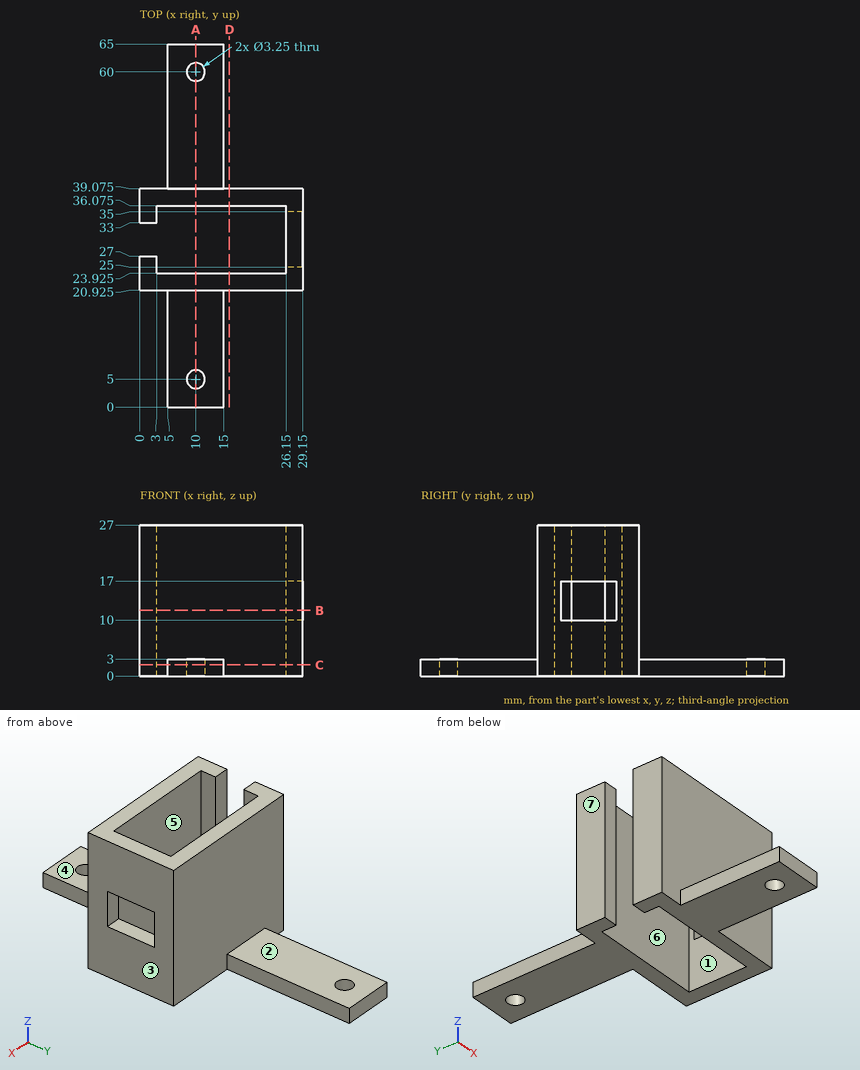
Input: dimensioned drawing with shaded views. Units: mm. Origin: part minimum x, y, z. A direction names the side the tool comes from. Coordinates: 2 decimals unless noted, no trailing zeros. Order: outer loops, then holes, each group sorted by start corner. A loop starts at its lowest first (then second) coordinate and runs counter-clockwise, first axis right, second up.
1. Cut plane B-B, the plane z = 11.75. Return loops of the section in (x, y) (3 decimals), plus the area to 3 significant figures.
Checked values:
outline: (0, 20.925) - (29.15, 20.925) - (29.15, 25) - (26.15, 25) - (26.15, 23.925) - (3, 23.925) - (3, 27) - (0, 27) - close; (0, 33) - (3, 33) - (3, 36.075) - (26.15, 36.075) - (26.15, 35) - (29.15, 35) - (29.15, 39.075) - (0, 39.075) - close
area: 200 mm2
2. Contact query for flat-ended pins moving along their axis: P1, Ø1.5, axis at x = 1.5, z = 9.5, coming from the +Y side (3 decimals); P2, Ø11.5, axis at x = 11, z = 10.5, coming from the -Y side (3 decimals); P3, Ø2.5, axis at y = 13, z = 1, coming from the +X side. Output: stop coordinate, or through.
Checked values:
P1: stops at y = 39.075
P2: stops at y = 20.925
P3: stops at x = 15
3. Cut plane C-C, the plane z = 2. Return loops of the section in (x, y) (3 decimals).
Checked values:
outline: (0, 20.925) - (5, 20.925) - (5, 0) - (15, 0) - (15, 20.925) - (29.15, 20.925) - (29.15, 39.075) - (15, 39.075) - (15, 65) - (5, 65) - (5, 39.075) - (0, 39.075) - (0, 33) - (3, 33) - (3, 36.075) - (26.15, 36.075) - (26.15, 23.925) - (3, 23.925) - (3, 27) - (0, 27) - close; hole circle Ø3.25 at (10, 5); hole circle Ø3.25 at (10, 60)
4. Draft query along X for the marked faces 4, 5, 6 and 7. Return one class per face: +X half, -X half, draft (parallel to the pull), parting line (faces both ways), or undercut.
Checked values:
face 4: draft
face 5: undercut
face 6: undercut
face 7: -X half
5. Access query for the marked faces 1, 2 and 3. Directions: +Z, -Z, +X, -X, +Y, -Y. A direction counts if a zero-diameter tool reaches every point of the face in a straight line with its end or side. Return the directions, or none.
Checked values:
face 1: +Z, -Z
face 2: +Z, +X, -X, +Y
face 3: +Z, -Z, +X, +Y, -Y
6. Cut plane D-D, the plane x = 16. Return loops of the section in (y, z) (3 decimals), plus the area to 3 significant figures.
Checked values:
outline: (20.925, 0) - (23.925, 0) - (23.925, 27) - (20.925, 27) - close; (36.075, 0) - (39.075, 0) - (39.075, 27) - (36.075, 27) - close
area: 162 mm2
7. Cut plane A-A, the plane x = 10. Return loops of the section in (y, z) (3 decimals), plus the area to 3 significant figures.
Checked values:
outline: (0, 0) - (3.375, 0) - (3.375, 3) - (0, 3) - close; (6.625, 0) - (23.925, 0) - (23.925, 27) - (20.925, 27) - (20.925, 3) - (6.625, 3) - close; (36.075, 0) - (58.375, 0) - (58.375, 3) - (39.075, 3) - (39.075, 27) - (36.075, 27) - close; (61.625, 0) - (65, 0) - (65, 3) - (61.625, 3) - close
area: 283 mm2
8. Ray query, line 1 along Y through (x, z) = (10, 2.4) (3 decimals); line 2 along Y through (x, z) = (3.5, 14.75) (3 decimals); line 3 along Y through (x, z) = (27.25, 10.5) (3 decimals). Return the intervals inside material, ascending.
Checked values:
line 1: y = 0 to 3.375, 6.625 to 23.925, 36.075 to 58.375, 61.625 to 65
line 2: y = 20.925 to 23.925, 36.075 to 39.075
line 3: y = 20.925 to 25, 35 to 39.075
